The model under review builds one solid part; all positions refer to its coordinate system, in mm. Face numbers are marked on the shaded views. A direction names the side the tool comes from. Round coordinates to 2 decimals unless told otherwise and drop trailing zeros. Write each loop counter-clockwise with the first axis right and the second up, starting at its lowest first coordinate (ties: lowest second). Pieces come first, ordered by that corner, then holes. Notation, with made-up numbers: M -2,54.25 L 7,54.25 A19 ccw 7,86.25 Z; hole C 76.5,-32.5 d4. An arc over 180 degrees is marked long. Write item = value, one per line. Start each with the question number.
Item 1: Take a section at B-B, the plane z = 0. Give the boundary of the cut face in (x, y) (3 decimals), plus the area to 3 significant figures.
Item 2: Take a section at A-A, the plane y = 0. Give the boundary of the cut face in (x, z) (3 decimals), plus the area to 3 significant figures.
Item 3: Take a section at C-C, the plane x = 134.5. Give the boundary of the cut face in (y, z).
Item 4: Take a section at D-D, the plane y = 10.5. Give the boundary of the cut face in (x, z), plus the area to 3 significant figures.
Item 5: For pin 1 Ø3 at (x, z) = (30.5, 4.5) entering from +Y; pin 2 Ø10 at (x, z) = (91, 3.5) entering from +Y; pin 3 Ø6 at (y, z) = (2, 8) entering from +X; pin 4 Ø2 at (x, z) = (66.5, 2) entering from -Y, all flat-tipped, find the tip position at first contact; note any pin that passes through.
Item 6: To check wall thickness, follow line 1 along X through (y, z) = (0, -1.5) (3 decimals); line 2 along Y through (x, z) = (146.05, 2.25) (3 decimals); line 3 along Y through (x, z) = (143.5, 0). State the ranges of each line that lie inside material, in increasing order.
Item 7: Tool access review of the marked faces 1 and 2: name each direction out of +Z, -Z, +X, -X, +Y, -Y from which nothing blocks a thin tool from reaching the whole face with its end or side.
Autodesk Inventor part; units mm, degrees
ref_plane "Work Plane3" through (152.4, 0, 0) normal (0, 0, -1) x (-1, 0, 0)
ref_plane "YZ Plane" through (0, 0, 0) normal (1, 0, 0) x (0, 1, 0)
ref_plane "XZ Plane" through (0, 0, 0) normal (0, 1, 0) x (-1, 0, 0)
sketch "Sketch1" plane through (0, 0, 0) normal (1, 0, 0) x (0, 1, 0)
  circle A0 centre (0, 0) radius 12.7
  dimension "d0" = 25.4
extrude "Extrusion1" add sketch "Sketch1" along normal blind 1.27
sketch "Sketch2" plane through (1.27, 0, 0) normal (1, 0, 0) x (0, 0, -1)
  circle A0 centre (0, 0) radius 6.35
  dimension "d3" = 12.7
extrude "Extrusion2" add sketch "Sketch2" along normal blind 151.13
sketch "Sketch3" plane through (152.4, 0, 0) normal (1, 0, 0) x (0, 0, -1)
  circle A0 centre (0, 0) radius 6.35
  circle A1 centre (0, 0) radius 6.35
  point P0 (-6.35, 0)
  point P1 (6.35, 0)
ref_plane "Work Plane3" through (152.4, 0, 0) normal (0, 0, -1) x (-1, 0, 0)
ref_plane "Work Plane1" through (152.4, 0, 6.35) normal (0, 0, 1) x (1, 0, 0)
ref_plane "Work Plane2" through (152.4, 0, -6.35) normal (0, 0, -1) x (-1, 0, 0)
sketch "Sketch4" plane through (152.4, 0, -6.35) normal (0, 0, -1) x (-1, 0, 0)
  circle A0 centre (6.35, 0) radius 3.175
  line L0 (0, 6.35) -> (0, -6.35)
  point P0 (152.4, 0)
  dimension "d6" = 6.35
  dimension "d7" = 6.35
extrude "Extrusion3" cut sketch "Sketch4" against normal blind 12.7
properties part number "Intake Basic Piston - Inner"
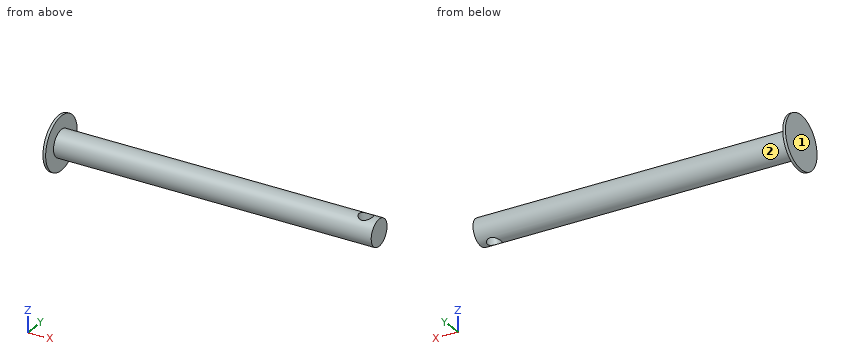
Response values:
q1.outline = M 0,-12.7 L 1.27,-12.7 L 1.27,-6.35 L 152.4,-6.35 L 152.4,6.35 L 1.27,6.35 L 1.27,12.7 L 0,12.7 Z; hole C 146.05,0 d6.35
q1.area = 1,920 mm2
q2.outline = M 0,-12.7 L 1.27,-12.7 L 1.27,-6.35 L 142.875,-6.35 L 142.875,6.35 L 1.27,6.35 L 1.27,12.7 L 0,12.7 Z; M 149.225,-6.35 L 152.4,-6.35 L 152.4,6.35 L 149.225,6.35 Z
q2.area = 1,870 mm2
q3.outline = C 0,0 d12.7
q4.outline = M 0,-7.14 L 1.27,-7.14 L 1.27,7.14 L 0,7.14 Z
q4.area = 18.1 mm2
q5.pin_1 = 5.6
q5.pin_2 = 6.35
q5.pin_3 = 152.4
q5.pin_4 = -6.27
q6.line_1 = 0 to 142.875, 149.225 to 152.4
q6.line_2 = -5.938 to -3.175, 3.175 to 5.938
q6.line_3 = -6.35 to -1.89, 1.89 to 6.35
q7.face_1 = +Z, -Z, -X, +Y, -Y
q7.face_2 = +X
